```python
from build123d import *

# Parameters (mm, degrees)
F0_W     = 50
F0_H     = 25
F1_DEPTH = 50
F2_R     = 4.6101
F3_DEPTH = 11.938
F3_TAPER = 2.5
F4_R     = 4.61
F5_DEPTH = 13.589
F5_TAPER = 8
F7_DEPTH = 2


with BuildPart() as f1:
    # F0 (on Front) → F1 (new body)
    with BuildSketch(Plane.XZ):
        with Locations((1.772807911, 0.3909162391)):
            Rectangle(F0_W, F0_H)
    extrude(amount=F1_DEPTH)

    # F2 (on face) → F3 (cut)
    with BuildSketch(Plane.XY.offset(12.8909162391)):
        with Locations((0, -29.7321814987)):
            Circle(F2_R)
    extrude(amount=-F3_DEPTH, taper=F3_TAPER, mode=Mode.SUBTRACT)

    # F4 (on face) → F5 (cut)
    with BuildSketch(Plane.XY.offset(12.8909162391)):
        with Locations((-11.7101902142, -14.4315985963)):
            Circle(F4_R)
    extrude(amount=-F5_DEPTH, taper=F5_TAPER, mode=Mode.SUBTRACT)

    # F6 (on face) → F7 (cut)
    with BuildSketch(Plane.XY.offset(12.8909162391)):
        Polygon((-20.116565749, -5.4274424911), (-20.116565749, -8.9698005468), (-18.6207834631, -8.9243609875), (-18.6207834631, -5.4274424911), (-18.6207834631, -4.2068846524), (-20.8131559193, -4.2068846524), (-20.8399798721, -5.4274424911), align=None)
        Polygon((8.8972449303, -23.4584081918), (8.8972449303, -21.9049714506), (8.8972449303, -20.8508521318), (6.0677705333, -20.8508521318), (6.0677705333, -21.9049714506), (7.6766866259, -21.9049714506), (7.6766866259, -22.6816888899), (6.2342090532, -22.6816888899), (6.2342090532, -25.6776046008), (8.8972449303, -25.6776046008), (8.8972449303, -24.6234852821), (7.2328480892, -24.6234852821), (7.2328480892, -23.4584081918), align=None)
    extrude(amount=-F7_DEPTH, mode=Mode.SUBTRACT)


solid = f1.part
```
The model under review builds one solid part; all positions refer to its coordinate system, in mm. A direction names the side the tool comes from. Round coordinates to 2 decimals unless told otherwise and drop trailing zeros. Write each loop counter-clockwise with the first axis right and the second up, starting at its lowest first coordinate (ties: lowest second). Pieces come first, ordered by that corner, then holes.
(1) We need section B-B on z = 9. Give the boundary of the cut face in (x, y), and give its area (3 significant figures).
(2) Wall thickness on L1, parallel to Y at x = 2, z = 9.25; L2, parallel to X at y = -28.5, z = 1; L3, parallel to Y at x = -3, z = 11: over which ranges is each line inside the solid? List them lowest first.
(3) Mouldability with a two-part tool opening along Y and no side actions: class faces 3 (the flat face through (8, -23.458, 12)), 4 (the flat face through (1, -50, 1)), 5 (the flat face through (26.773, -25, 0)) as +Y half, -Y half, draft (parallel to the pull), parting line (faces both ways), or undercut.
(4) Machinability: for faces 1 (the flat face through (0, -30, 0.953)), 2 (the flat face through (-23.227, -25, 0)), which of the approach directions +Z, -Z, +X, -X, +Y, -Y give a long, thin tool a straight path to every point of the face, cutting with its end or side? Answer none if there is none.
(5) Insertion check: pin 1 (5 mm diameter, centred on x = 3.5, y = -32.5, fed in from +Z). The pin has a flat end and moves straight along its axis. Give the tip position at first contact, or say it passes through.
(6) We need section A-A on x = 0. Give the boundary of the cut face in (y, z), and give its area (3 significant figures).
Findings below:
1. outline: (-23.23, -50) - (26.77, -50) - (26.77, 0) - (-23.23, 0) - close; hole circle Ø8.13 at (-11.71, -14.43); hole circle Ø8.88 at (0, -29.73)
1. area: 2,390 mm2
2. L1: y = -50 to -33.71, -25.76 to 0
2. L2: x = -23.23 to -3.9, 3.9 to 26.77
2. L3: y = -50 to -33.12, -26.34 to 0
3. face 3: undercut
3. face 4: -Y half
3. face 5: draft
4. face 1: +Z
4. face 2: +Z, -Z, -X, +Y, -Y
5. pin 1: stops at z = 12.89
6. outline: (-50, -12.11) - (0, -12.11) - (0, 12.89) - (-25.12, 12.89) - (-25.64, 0.95) - (-33.82, 0.95) - (-34.34, 12.89) - (-50, 12.89) - close
6. area: 1,150 mm2
